Here's how the part is built. I have some questions about the finished solid (model axes, mm). Coordinates: 2 decimals unless noted, no trailing zeros. Write each loop counter-clockwise with the first axis right and the second up, starting at its lowest first coordinate (ties: lowest second). Pieces come first, ordered by that corner, then holes. Notation, with made-up numbers: M 53.5,43 L 62.5,43 A16 ccw 62.5,69 Z; hole C 25.25,83 d11. An arc over 180 degrees is marked long. Use a Markdown table: item, result.
```python
from build123d import *

# Parameters (mm, degrees)
BASE_FLANGE1_DEPTH = 3.175
FILLET1_R          = 10


# Sheet-metal steps are written as plain solids
with BuildPart() as part:
    # Sketch2 → Base-Flange1 (new body)
    with BuildSketch(Plane.XY):
        Polygon((-1276.361705331, -175.10923744), (-1276.361705331, 175.10923744), (-944.783937855, 175.10923744), (0, 302.529477003), (0, -302.529477003), (-944.783937855, -175.10923744), align=None)
    extrude(amount=-BASE_FLANGE1_DEPTH)

    # Fillet1
    fillet1_edges = [part.edges().sort_by_distance(p)[0] for p in [
        (0, 302.529477003, -1.5875),
        (0, -302.529477003, -1.5875),
        (-944.783937855, -175.10923744, -1.5875),
        (-1276.361705331, -175.10923744, -1.5875),
        (-1276.361705331, 175.10923744, -1.5875),
    ]]
    fillet(fillet1_edges, radius=FILLET1_R)


solid = part.part
```
1. Suppose I cut it at A-A on z = -1.1. Write out the boundary of the cut face in (x, y).
Answers follow:
| item | result |
|---|---|
| outline | M -1276.36,-165.11 A10 ccw -1266.36,-175.11 L -945.46,-175.11 A10 cw -944.12,-175.2 L -11.34,-301 A10 ccw 0,-291.09 L 0,291.09 A10 ccw -11.34,301 L -944.78,175.11 L -1266.36,175.11 A10 ccw -1276.36,165.11 Z |
2. I need wall thicknesses on probe 1 along X at (y, z) = (-166.5, -1.4); probe 2 along Y at (x, z) = (-1078, -0.15); probe 3 along Y at (x, z) = (-508, -2.1). Which ranges of each line are inside material? Lowest first, please.
Answers follow:
| item | result |
|---|---|
| probe 1 | x = -1276.26 to 0 |
| probe 2 | y = -175.11 to 175.11 |
| probe 3 | y = -234.02 to 234.02 |
3. Suppose I cut it at B-B on x = -987.5. Write out the boundary of the cut face in (y, z) (3 decimals).
Answers follow:
| item | result |
|---|---|
| outline | M -175.109,-3.175 L 175.109,-3.175 L 175.109,0 L -175.109,0 Z |
4. Suppose I cut it at C-C on y = -259. Write out the boundary of the cut face in (x, z) (3 decimals), and give its area (3 significant figures).
Answers follow:
| item | result |
|---|---|
| outline | M -322.758,-3.175 L 0,-3.175 L 0,0 L -322.758,0 Z |
| area | 1,020 mm2 |
5. Will these pins go through, and if not, where does the flat tip stop? pin 1 Ø1 at (x, z) = (-182.5, -2.5) entering from -Y; pin 2 Ø1 at (x, y) = (-996.5, 19) entering from +Z.
Answers follow:
| item | result |
|---|---|
| pin 1 | stops at y = -277.98 |
| pin 2 | stops at z = 0 |
